CAD build for the part. Positions are in the model's coordinates, mm. A direction names the side the tool comes from. Round coordinates to 2 decimals unless told otherwise and drop trailing zeros. Loops run counter-clockwise (first coordinate to the right, second up) from the corner with the lowest first, then second, coordinate; pieces in that order, holes last. Notation, with made-up numbers: (-31.75, 10) -> (16.25, 10) arc R24 ccw to (16.25, 40) -> close; hole circle Ø9 at (63.5, -23). An arc over 180 degrees is marked (long way). Answer as CSV lines item,"result".
```python
from build123d import *

# Parameters (mm, degrees)
F0_W      = 50
F0_H      = 50
F1_DEPTH  = 50
F3_DEPTH  = 10
F4_R      = 25
F5_DEPTH  = 20
F11_DEPTH = 10


with BuildPart() as f1:
    # F0 (on Top) → F1 (new body)
    with BuildSketch(Plane.XY):
        with Locations((25, 25)):
            Rectangle(F0_W, F0_H)
    extrude(amount=F1_DEPTH)

    # F2 (on face) → F3 (cut)
    with BuildSketch(Plane.XY.offset(50)):
        with BuildLine():
            ThreePointArc((0, 15), (-10.6066017178, -10.6066017178), (15, 0))
            Line((15, 0), (0, 0))
            Line((0, 0), (0, 15))
        make_face()
        with BuildLine():
            ThreePointArc((0, 15), (10.6066017178, 10.6066017178), (15, 0))
            Line((15, 0), (25, 0))
            Line((25, 0), (25, 15.000000596))
            Line((25, 15.000000596), (15, 25))
            Line((15, 25), (0, 25))
            Line((0, 25), (0, 15))
        make_face()
    extrude(amount=-F3_DEPTH, mode=Mode.SUBTRACT)

    # F4 (on face) → F5 (cut)
    with BuildSketch(Plane(origin=(0, 0, 0), x_dir=(1, 0, 0), z_dir=(0, 0, -1))):
        Circle(F4_R)
    extrude(amount=-F5_DEPTH, mode=Mode.SUBTRACT)

    # F6 (on face) → F7 (revolve, cut)
    with BuildSketch(Plane.XZ):
        Polygon((25, 20), (0, 50), (0, 20), align=None)
    revolve(axis=Axis((0, 0, 35), (0, 0, -1)), mode=Mode.SUBTRACT)

    # F10 (on offset) → F11 (cut, through all)
    with BuildSketch(Plane.YZ.offset(44)):
        Polygon((0, 50), (0, 10), (30, 10), (30, 20), (40, 20), (40, 50), align=None)
        with BuildLine():
            Line((30, 20), (30, 10))
            ThreePointArc((30, 10), (37.0710678119, 12.9289321881), (40, 20))
            Line((40, 20), (30, 20))
        make_face()
    extrude(amount=-F11_DEPTH, mode=Mode.SUBTRACT)


solid = f1.part
```
Q1. Slice it at C-C, the plane y = 36.5. Give the cut face in (x, z).
Results:
outline,"(0, 0) -> (50, 0) -> (50, 50) -> (44, 50) -> (44, 12.4) -> (34, 12.4) -> (34, 50) -> (0, 50) -> close"
Q2. Two-plate mould, pull along X, no slides. Class faces 4 (the flat face through (39, 15, 10)), 5 (the flat face through (50, 25, 25)), 6 (the flat face through (0, 36, 25)), 7 (the flat face through (25, 50, 25)): pulls with the +X half, pulls with the -X half, needs draft (parallel to the pull), parting line crosses it, or undercut.
Results:
face 4,"undercut"
face 5,"pulls with the +X half"
face 6,"pulls with the -X half"
face 7,"needs draft"
Q3. Slice it at D-D, the plane z = 38. Give the cut face in (x, y), and give its area (3 significant figures).
Results:
outline,"(0, 10) arc R10 cw to (10, 0) -> (34, 0) -> (34, 40) -> (44, 40) -> (44, 0) -> (50, 0) -> (50, 50) -> (0, 50) -> close"
area,"2,020 mm2"
Q4. Slice it at B-B, the plane x = 41. Give the cut face in (y, z).
Results:
outline,"(0, 0) -> (50, 0) -> (50, 50) -> (40, 50) -> (40, 20) arc R10 cw to (30, 10) -> (0, 10) -> close"
Q5. Drop flat-ended pins along their axis: pin 1 Ø5 at (x, z) = (40, 38.5) entering from -Y; pin 2 Ø3 at (y, z) = (20.5, 45) entering from -X. Give the stop position or say it passes through.
Results:
pin 1,"y = 40"
pin 2,"x = 18"
Q6. Tool access for faces 1 (the flat face through (44, 20, 30)), 2 (the flat face through (15, 15, 40)), 3 (the flat face through (8, 25, 45)): list every direction of +Z, -Z, +X, -X, +Y, -Y with a clear straight run to the whole face (end or side of a thin tool).
Results:
face 1,"+Z, -Y"
face 2,"+Z"
face 3,"+Z, -X"
Q7. Probe L1, parallel to X at y = 39, z = 24; L2, parallel to Y at x = 20, z = 16; L3, parallel to Y at x = 35.5, z = 39. List the from-to ranges inside material, lowest first. Write a range as [from, to].
Results:
L1,"[0, 34], [44, 50]"
L2,"[15, 50]"
L3,"[40, 50]"
Q8. Slice it at A-A, the plane z = 26. Give the cut face in (x, y), and give its area (3 significant figures).
Results:
outline,"(0, 20) arc R20 cw to (20, 0) -> (34, 0) -> (34, 40) -> (44, 40) -> (44, 0) -> (50, 0) -> (50, 50) -> (0, 50) -> close"
area,"1,790 mm2"
